Could you check a few things on this model? Use its own coordinates, in mm. Round coordinates to 2 decimals unless told otherwise and drop trailing zeros. Write each loop counter-clockwise with the first axis right and the second up, starting at its lowest first coordinate (ties: lowest second). Pieces come first, ordered by that corner, then holes. Notation, with made-up numbers: (12.5, 59) - (63.5, 59) arc R25 cw to (63.5, 76) - close; hole circle Ø5 at (-19, -29). An arc over 180 degrees is marked (long way). Write each question's results on one line, items separated by ' | '. Start each with the question number.
(1) Thinking about a two-plate mould opening in Y: for faces 1 (the flat face through (5.1, 25.1, 0.5)), 2 (the flat face through (5.1, 4.9, 0.5)), 3 (the cylindrical face through (23.87, 19.77, 0.49)), which applies, +Y half, -Y half, draft (parallel to the pull), parting line (faces both ways), or undercut?
(2) Imagine slicing it at B-B on z = 0.6. State how many separate pieces and enclosed holes the cut face has, then the cut area to 3 significant figures.
(3) Please list where these lines run through material, in increasing order: line 1 (Y direction, x = 207.5, z = 0.55); line 2 (Y direction, x = 195, z = 0.2); line 3 (Y direction, x = 112.5, z = 0.7). Write a range as [from, to].
(4) Imagine slicing it at A-A on x = 45. Write out the boundary of the cut face in (y, z), then the cut area to 3 significant figures.
```python
from build123d import *

# Parameters (mm, degrees)
SKETCH_1_W          = 240
SKETCH_1_H          = 75
EXTRUDE_1_DEPTH     = 1
CUT_EXTRUDE_2_DEPTH = 10
SKETCH_4_W          = 80
SKETCH_4_H          = 45
CUT_EXTRUDE_3_DEPTH = 10
CHAMFER_1_SIZE      = 10
SKETCH_5_R          = 1.6
SKETCH_5_R_2        = 2.1
CUT_EXTRUDE_4_DEPTH = 10
EXTRUDE_2_DEPTH     = 1


with BuildPart() as part:
    # 草图1 → 凸台-拉伸1 (new body)
    with BuildSketch(Plane.XY):
        with Locations((120, 37.5)):
            Rectangle(SKETCH_1_W, SKETCH_1_H)
    extrude(amount=EXTRUDE_1_DEPTH)

    # 草图3 → 切除-拉伸2 (cut)
    with BuildSketch(Plane(origin=(0, 0, 0), x_dir=(-1, 0, 0), z_dir=(0, 0, -1))):
        Polygon((-130, 7.679491924), (-110, 7.679491924), (-100, 25), (-110, 42.320508076), (-130, 42.320508076), (-140, 25), align=None)
        Polygon((-148.469655115, 56.990381057), (-135, 33.660254038), (-130, 42.320508076), (-110, 42.320508076), (-105, 33.660254038), (-91.530344885, 56.990381057), (-95, 63), (-145, 63), align=None)
    extrude(amount=-CUT_EXTRUDE_2_DEPTH, mode=Mode.SUBTRACT)

    # 草图4 → 切除-拉伸3 (cut)
    with BuildSketch(Plane(origin=(0, 0, 0), x_dir=(-1, 0, 0), z_dir=(0, 0, -1))):
        with Locations((-40, 52.5)):
            Rectangle(SKETCH_4_W, SKETCH_4_H)
    extrude(amount=-CUT_EXTRUDE_3_DEPTH, mode=Mode.SUBTRACT)

    # 倒角1
    chamfer_1_edges = [part.edges().sort_by_distance(p)[0] for p in [
        (80, 75, 0.5),
        (0, 30, 0.5),
        (80, 30, 0.5),
        (240, 75, 0.5),
        (240, 0, 0.5),
        (0, 0, 0.5),
    ]]
    chamfer(chamfer_1_edges, length=CHAMFER_1_SIZE)

    # 草图5 → 切除-拉伸4 (cut)
    with BuildSketch(Plane(origin=(0, 0, 0), x_dir=(-1, 0, 0), z_dir=(0, 0, -1))):
        with Locations((-5, 15)):
            Circle(SKETCH_5_R)
        with Locations((-195, 12)):
            Circle(SKETCH_5_R_2)
        with Locations((-45, 12)):
            Circle(SKETCH_5_R_2)
        with Locations((-235, 37.5)):
            Circle(SKETCH_5_R)
        with Locations((-207.5, 68)):
            Circle(SKETCH_5_R)
        with Locations((-192.5, 68)):
            Circle(SKETCH_5_R)
        with Locations((-127.5, 68)):
            Circle(SKETCH_5_R)
        with Locations((-112.5, 68)):
            Circle(SKETCH_5_R)
        with Locations((-25, 18)):
            Circle(SKETCH_5_R_2)
    extrude(amount=-CUT_EXTRUDE_4_DEPTH, mode=Mode.SUBTRACT)

    # 草图6 → 凸台-拉伸2 (add)
    with BuildSketch(Plane(origin=(0, 0, 0), x_dir=(-1, 0, 0), z_dir=(0, 0, -1))):
        Polygon((-135, 33.660254038), (-123.469655115, 13.689110868), (-116.530344885, 13.689110868), (-105, 33.660254038), (-100, 25), (-110, 7.679491924), (-130, 7.679491924), (-140, 25), align=None)
    extrude(amount=-EXTRUDE_2_DEPTH)


solid = part.part
```
Response:
1) face 1: +Y half | face 2: -Y half | face 3: undercut
2) separate pieces: 1 | enclosed holes: 10 | area: 12,400 mm²
3) line 1: [0, 66.4], [69.6, 75] | line 2: [0, 9.9], [14.1, 75] | line 3: [0, 20.67], [63, 66.4], [69.6, 75]
4) outline: (0, 0) - (9.9, 0) - (9.9, 1) - (0, 1) - close; (14.1, 0) - (30, 0) - (30, 1) - (14.1, 1) - close | area: 25.8 mm²
